Source: three-view drawing plus pictorial views. Frame: mm from the lowest corner of the part. A direction names the side the tool comes from. Give positions to 0.01 mm unless a question says otherwise; leave off trailing zeros. Loops run counter-clockwise (first coordinate to the right, second up) from the corner with the lowest first, then second, coordinate; pieces in that order, holes last. Notation, with made-up numbers: M 54.5,46.5 L 111.5,46.5 A21 cw 111.5,68.5 Z; hole C 36.25,21 d8. An arc over 180 degrees is marked long. Answer as a JSON object with one key per item and string values. Group by question number.
1) Section query B-B on z = 29. Return loops of the section in (x, y).
2) First-contact query: P1, Ø1.5, axis at y = 3.5, z = 13, coming from the +X side; P2, Ø1.5, axis at x = 33.5, z = 8.5, coming from the -Y side. Flat tips, straight axial feed; report the tip coordinate or a pass-through.
3) Section query A-A on x = 21.5. Return loops of the section in (y, z), plus the area to 3 significant figures.
4) Access query for the marked faces 1 and 2. Directions: +Z, -Z, +X, -X, +Y, -Y. A direction counts if a zero-diameter tool reaches every point of the face in a straight line with its end or side. Return the directions, or none.
5) Section query C-C on y = 23.25. Return loops of the section in (x, z).
6) Ray query, L1, parallel to X at y = 2.25, z = 11.5; L2, parallel to Z at x = 19, y = 24; L3, parallel to Z at x = 24.5, y = 3 (1 decimal). Return the intervals inside material, ascending.
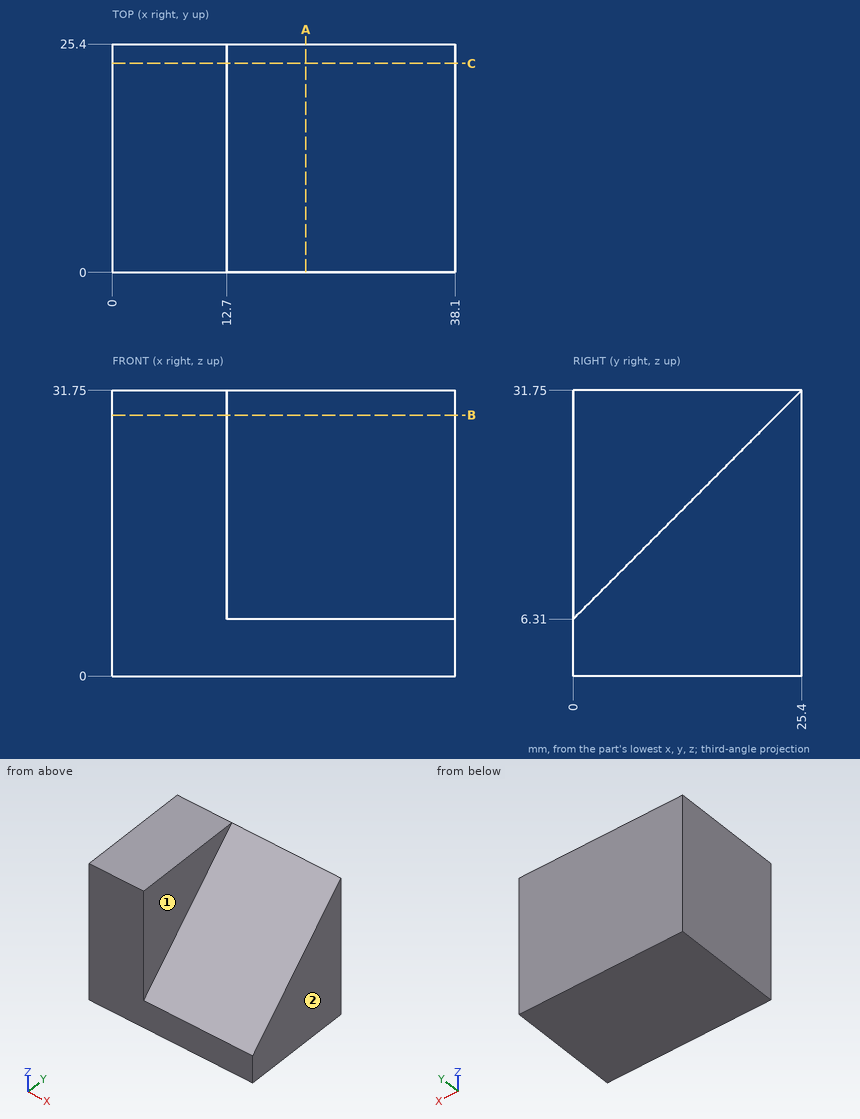
Output:
{
 "1": {"outline": "M 0,0 L 12.7,0 L 12.7,22.65 L 38.1,22.65 L 38.1,25.4 L 0,25.4 Z"},
 "2": {"P1": "stops at x = 12.7", "P2": "stops at y = 1.44"},
 "3": {"outline": "M 0,0 L 25.4,0 L 25.4,31.75 L 0,6.31 Z", "area": "483 mm^2"},
 "4": {"face 1": "+Z, +X, -Y", "face 2": "+Z, -Z, +X, +Y, -Y"},
 "5": {"outline": "M 0,0 L 38.1,0 L 38.1,29.6 L 12.7,29.6 L 12.7,31.75 L 0,31.75 Z"},
 "6": {"L1": "x = 0 to 12.7", "L2": "z = 0 to 30.35", "L3": "z = 0 to 9.3"}
}
